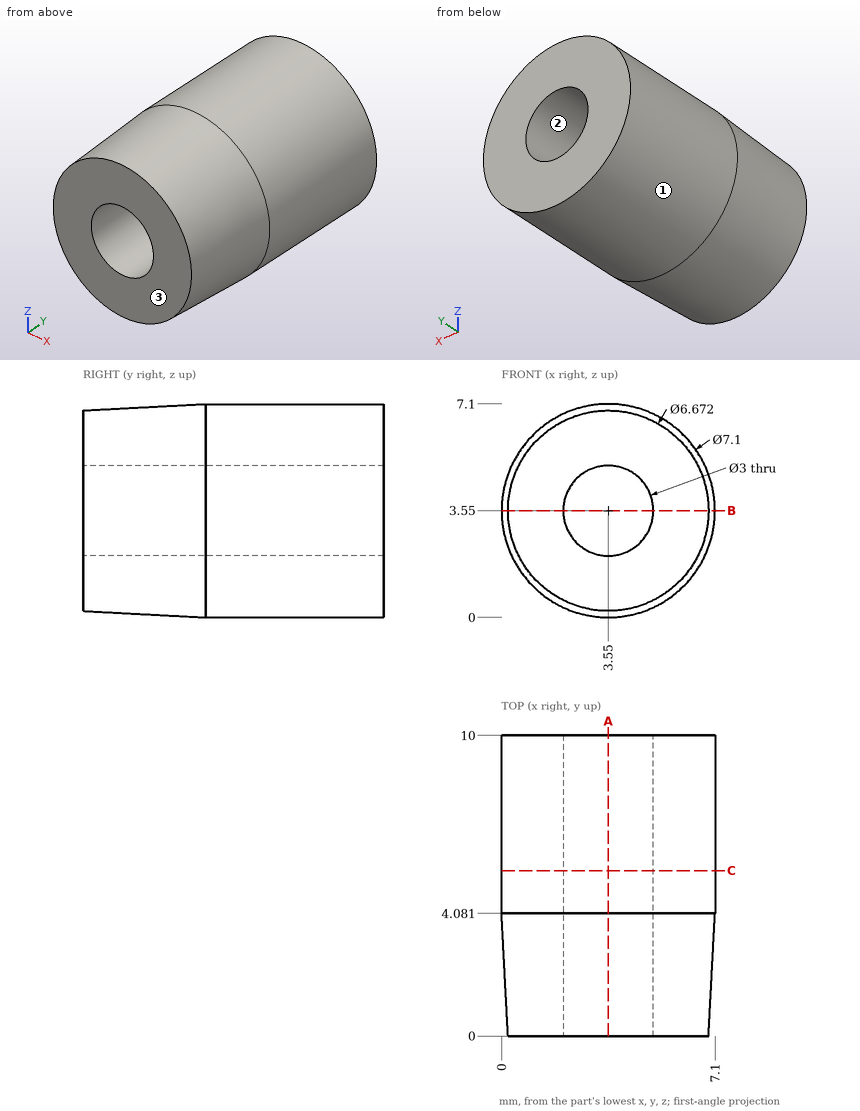
Can you work these out from the drawing? Everything is in mm from the part's minimum corner. Round coordinates to 2 decimals unless told otherwise and drop trailing zeros. Loops run counter-clockwise (first coordinate to the right, second up) from the corner with the lowest first, then second, coordinate; pieces in that order, holes last. Notation, with made-up numbers: (16, 78) - (55, 78) arc R18 ccw to (55, 83) - close; hole circle Ø9 at (-12, -36.5). An arc over 180 degrees is marked (long way). Answer in a Markdown table with one row per item. Add a question column.
(1) If we section it at C-C (y = 5.5): Please give me the cut outline in (x, z).
(2) I need wall thicknesses on line 1 along Z through (x, y) = (3.55, 6.5); line 2 along Z through (x, y) = (2.75, 8.25). Which ranges of each line are inside material? Lowest first, please.
(3) If we section it at A-A (x = 3.55): Please give me the cut outline in (y, z).
(4) I'm going to push flat-ended pins straight in: pin 1 (3 mm diameter, centred on x = 2.5, z = 4.5, fed in from +Y); pin 2 (3 mm diameter, centred on x = 4.5, y = 2.5, fed in from +Z); pin 3 (3 mm diameter, centred on y = 5, z = 6, fed in from -X); pin 4 (2.5 mm diameter, centred on x = 3.55, z = 3.55, fed in from +Y). Where does each tip first touch, or does it pass through?
(5) If we section it at B-B (z = 3.55): Please give me the cut outline in (x, y), plus the area to 3 significant figures.
(6) If we mould it in two halves opening along Z, with no side actions, what happens to the marked faces 1, 2 and 3? For each: pulls with the +Z half, pulls with the -Z half, needs draft (parallel to the pull), parting line crosses it, or undercut.
Model answer:
| question | item | result |
|---|---|---|
| 1 | outline | circle Ø7.1 at (3.55, 3.55); hole circle Ø3 at (3.55, 3.55) |
| 2 | line 1 | z = 0 to 2.05, 5.05 to 7.1 |
| 2 | line 2 | z = 0.09 to 2.28, 4.82 to 7.01 |
| 3 | outline | (0, 0.21) - (4.08, 0) - (10, 0) - (10, 2.05) - (0, 2.05) - close; (0, 5.05) - (10, 5.05) - (10, 7.1) - (4.08, 7.1) - (0, 6.89) - close |
| 4 | pin 1 | stops at y = 10 |
| 4 | pin 2 | stops at z = 7.08 |
| 4 | pin 3 | stops at x = 0.13 |
| 4 | pin 4 | passes through |
| 5 | outline | (0, 4.08) - (0.21, 0) - (2.05, 0) - (2.05, 10) - (0, 10) - close; (5.05, 0) - (6.89, 0) - (7.1, 4.08) - (7.1, 10) - (5.05, 10) - close |
| 5 | area | 40.1 mm² |
| 6 | face 1 | parting line crosses it |
| 6 | face 2 | undercut |
| 6 | face 3 | needs draft |
